Part model, mm, in its own coordinate system. A direction names the side the tool comes from. Round coordinates to 2 decimals unless told otherwise and drop trailing zeros. Loops run counter-clockwise (first coordinate to the right, second up) from the corner with the lowest first, then second, coordinate; pieces in that order, holes last. Notation, with made-up numbers: M -7.75,39.25 L 14.25,39.25 A20 ccw 14.25,50.25 Z; hole C 42,23.25 d5. An arc over 180 degrees is marked long. Write each question's results on one line, items separated by ' | '.
from build123d import *

# Parameters (mm, degrees)
SKETCH1_W           = 50
SKETCH1_H           = 50
BOSS_EXTRUDE1_DEPTH = 10
SKETCH2_R           = 22
BOSS_EXTRUDE2_DEPTH = 21
BOSS_EXTRUDE3_DEPTH = 18
SKETCH4_R           = 4.5
CUT_EXTRUDE1_DEPTH  = 87.029064856
BOSS_EXTRUDE4_START = -9
SKETCH6_W           = 8
SKETCH6_H           = 15
BOSS_EXTRUDE4_DEPTH = 32
BOSS_EXTRUDE5_DEPTH = 36
SKETCH12_R          = 4.5
CUT_EXTRUDE2_DEPTH  = 48
FILLET1_R           = 3
FILLET2_R           = 3


with BuildPart() as part:
    # Sketch1 → Boss-Extrude1 (new body)
    with BuildSketch(Plane.XY):
        with Locations((25, 25)):
            Rectangle(SKETCH1_W, SKETCH1_H)
    extrude(amount=BOSS_EXTRUDE1_DEPTH)

    # Sketch2 → Boss-Extrude2 (add)
    with BuildSketch(Plane.XY.offset(10)):
        with Locations(Location((25, 25, 0), (0, 0, 180))):
            Circle(SKETCH2_R)
    extrude(amount=BOSS_EXTRUDE2_DEPTH)

    # Sketch3 → Boss-Extrude3 (add)
    with BuildSketch(Plane.XY.offset(31)):
        Polygon((25, 11), (37.124355653, 18), (37.124355653, 32), (25, 39), (12.875644347, 32), (12.875644347, 18), align=None)
    extrude(amount=BOSS_EXTRUDE3_DEPTH)

    # Sketch4 → Cut-Extrude1 (cut, through all)
    with BuildSketch(Plane.XY.offset(49)):
        with Locations((25, 25)):
            Circle(SKETCH4_R)
    extrude(amount=-CUT_EXTRUDE1_DEPTH, mode=Mode.SUBTRACT)

    # Sketch6 → Boss-Extrude4 (add)
    with BuildSketch(Plane.XZ.offset(BOSS_EXTRUDE4_START)):
        with Locations((6, 17.5)):
            Rectangle(SKETCH6_W, SKETCH6_H)
    extrude(amount=-BOSS_EXTRUDE4_DEPTH)

    # Sketch10 → Boss-Extrude5 (add)
    with BuildSketch(Plane(origin=(73, 0, 0), x_dir=(0, 0, -1), z_dir=(1, 0, 0))):
        Polygon((-4, 16.917096231), (-4, 33.082903769), (-18, 41.165807537), (-32, 33.082903769), (-32, 16.917096231), (-18, 8.834192463), align=None)
    extrude(amount=-BOSS_EXTRUDE5_DEPTH)

    # Sketch12 → Cut-Extrude2 (cut)
    with BuildSketch(Plane(origin=(73, 0, 0), x_dir=(0, 0, -1), z_dir=(1, 0, 0))):
        with Locations((-18, 25)):
            Circle(SKETCH12_R)
    extrude(amount=-CUT_EXTRUDE2_DEPTH, mode=Mode.SUBTRACT)

    # Fillet1
    fillet1_edges = [part.edges().sort_by_distance(p)[0] for p in [
        (3, 25, 31),
    ]]
    fillet(fillet1_edges, radius=FILLET1_R)

    # Fillet2
    fillet2_edges = [part.edges().sort_by_distance(p)[0] for p in [
        (0, 50, 5),
        (50, 50, 5),
        (50, 0, 5),
        (0, 0, 5),
    ]]
    fillet(fillet2_edges, radius=FILLET2_R)


solid = part.part
Item 1: Band-saw the part on A-A on y = 25. Give the cut face in (x, z), and give its area (3 significant figures).
Filled sheet:
outline: M 0,0 L 20.5,0 L 20.5,49 L 12.88,49 L 12.88,31 L 6,31 A3 ccw 3,28 L 3,25 L 2,25 L 2,10 L 0,10 Z; M 29.5,0 L 50,0 L 50,4 L 73,4 L 73,13.5 L 29.5,13.5 Z; M 29.5,22.5 L 73,22.5 L 73,32 L 37.12,32 L 37.12,49 L 29.5,49 Z | area: 1,760 mm^2
Item 2: Band-saw the part on B-B on x = 52. Give the cut face in (y, z).
Filled sheet:
outline: M 8.83,18 L 16.92,4 L 33.08,4 L 41.17,18 L 33.08,32 L 16.92,32 Z; hole C 25,18 d9
Item 3: Band-saw the part on D-D on z = 26. Give the cut face in (x, y), and give its area (3 significant figures).
Filled sheet:
outline: M 43.73,13.45 L 73,13.45 L 73,36.55 L 43.73,36.55 A22 ccw long Z; hole C 25,25 d9 | area: 2,080 mm^2
Item 4: Wall check: L1, parallel to Y at x = 25, z = 15; L2, parallel to Z at x = 45, y = 25; L3, parallel to Z at x = 59, y = 25. Give the ranges that are in metal, low to high.
Filled sheet:
L1: 3 to 20.5, 29.5 to 47 | L2: 0 to 13.5, 22.5 to 32 | L3: 4 to 13.5, 22.5 to 32
Item 5: Which spindle directions (+Z, -Z, +X, -X, +Y, -Y) get a long thin tool onto all of the face, cutting with end or side? Do faces 1 (the flat face through (6, 9, 18)), 2 (the flat face through (37.124, 25, 40)), 3 (the flat face through (2.4, 24.8, 25)). Say none if no direction does.
Filled sheet:
face 1: +Z, -X, -Y | face 2: +Z, +X, +Y, -Y | face 3: +Z, -X
Item 6: Drop flat-ended pins along their axis: P1, Ø7.5, axis at y = 24, z = 14, coming from the -X side; P2, Ø13, axis at x = 66, y = 21, coming from the -Z side; P3, Ø8, axis at x = 17, z = 42, coming from the -Y side; P4, Ø5.5, axis at x = 25, y = 25, coming from the +Z side. Give the stop position or say it passes through.
Filled sheet:
P1: x = 2 | P2: z = 4 | P3: y = 13.31 | P4: through
Item 7: Band-saw the part on C-C on z = 36.5. Give the cut face in (x, y), and give its area (3 significant figures).
Filled sheet:
outline: M 12.88,18 L 25,11 L 37.12,18 L 37.12,32 L 25,39 L 12.88,32 Z; hole C 25,25 d9 | area: 446 mm^2
Item 8: Two-plate mould, pull along Z, no slides. Class faces 4 (the cylindrical face through (49.336, 26.352, 13.708)), 5 (the cylindrical face through (39.95, 8.86, 18.87)), 6 (the flat face through (19, 25, 0)), 7 (the flat face through (0, 25, 5)): +Z half, -Z half, draft (parallel to the pull), parting line (faces both ways), or undercut.
Filled sheet:
face 4: undercut | face 5: undercut | face 6: -Z half | face 7: draft
